Input: part model. Units: mm. Frame: model coordinates. Give positions to 0.01 mm unless a question says otherwise; leave off trailing zeros. Write each loop counter-clockwise with the first axis right and the second up, starting at its lowest first coordinate (ties: lowest second). Pieces come first, ordered by that corner, then holes. Notation, with made-up numbers: (63.5, 7.5) -> (97.5, 7.5) arc R22 cw to (97.5, 27.5) -> close; hole circle Ø4 at (66, -29.5). An arc over 180 degrees is marked (long way). Return JSON: item names as keys, results as strings. Group by question number.
Item 1: Pin query (flat end, axial travel): P1, Ø6, axis at x = 957.5, y = 88, coming from the +Z side; P2, Ø5.5, axis at x = 471.5, y = 84.5, coming from the -Z side; P3, Ø1.5, axis at x = 312.5, y = 76.5, coming from the +Z side; P4, Ø10, axis at x = 337, y = 73.5, coming from the -Z side. Return the tip coordinate at first contact, or that it passes through.
Item 2: Section B-B, the plane z = 16.25. Return loops of the section in (x, y).
Item 3: Line query: line 1 (Y direction, x = 1110, z = 4.5); line 2 (Z direction, x = 526.5, y = 73.5); line 3 (Y direction, x = 307, z = 1). Output: solid intervals per line, ascending. Write a range as [from, to].
Item 4: Section A-A, the plane x = 1159. Return loops of the section in (y, z).
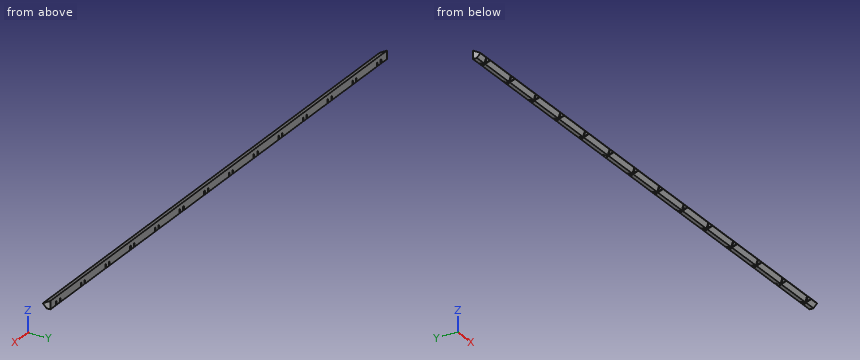
from build123d import *

# Parameters (mm, degrees)
PAD007_DEPTH           = 1500
POCKET004_DEPTH        = 11
LINEARPATTERN001_COUNT = 14
LINEARPATTERN001_PITCH = 110


with BuildPart() as part:
    # Sketch011 → Pad007 (new body)
    with BuildSketch(Plane.YZ):
        Polygon((92, 0), (81, 0), (71, 10), (71, 11), (92, 23.124356), align=None)
    extrude(amount=PAD007_DEPTH)

    # Sketch012 → Pocket004 (cut)
    with BuildSketch(Plane.XY):
        Polygon((6.70945, 46.612398), (8.29055, 45.387602), (35, 79.867074), (88.735058, 10.5), (78.064124, -3.275205), (79.645224, -4.5), (90, 8.867074), (100.354776, -4.5), (101.935876, -3.275205), (91.264942, 10.5), (118.29055, 45.387602), (116.70945, 46.612398), (90, 12.132926), (36.264942, 81.5), (46.935876, 95.275205), (45.354776, 96.5), (35, 83.132926), (24.645224, 96.5), (23.064124, 95.275205), (33.735058, 81.5), align=None)
    pocket004 = extrude(amount=POCKET004_DEPTH, mode=Mode.SUBTRACT)

    # LinearPattern001: Pocket004 ×14
    with Locations(*[(i * LINEARPATTERN001_PITCH, 0, 0) for i in range(1, LINEARPATTERN001_COUNT)]):
        add(pocket004, mode=Mode.SUBTRACT)


solid = part.part
Answer below:
{
 "1": {"P1": "stops at z = 22.55", "P2": "stops at z = 0", "P3": "stops at z = 14.61", "P4": "stops at z = 2.5"},
 "2": {"outline": "(0, 80.09) -> (1500, 80.09) -> (1500, 92) -> (0, 92) -> close"},
 "3": {"line 1": "y = [76.5, 92]", "line 2": "z = [7.5, 12.44]", "line 3": "y = [80, 92]"},
 "4": {"outline": "(71, 10) -> (81, 0) -> (92, 0) -> (92, 23.12) -> (71, 11) -> close"}
}
